from build123d import *

# Parameters (mm, degrees)
SKETCH_2_W          = 350
SKETCH_2_H          = 200
EXTRUDE_1_DEPTH     = 150
SHELL_1_T           = -20
CUT_EXTRUDE_1_REACH = 426.016
SKETCH_3_R          = 5
CUT_EXTRUDE_2_REACH = 426.016
SKETCH_4_R          = 7.5
CUT_EXTRUDE_3_REACH = 424.637


with BuildPart() as part:
    # 草图2 → 凸台-拉伸1 (new body)
    with BuildSketch(Plane(origin=(0, 0, 0), x_dir=(1, 0, 0), z_dir=(0, 1, 0))):
        with Locations((165.766338514, -86.518854231)):
            Rectangle(SKETCH_2_W, SKETCH_2_H)
    extrude(amount=EXTRUDE_1_DEPTH)

    # 抽壳1
    shell_1_openings = [part.faces().sort_by_distance(p)[0] for p in [
        (165.766338514, 150, 86.518854231),
    ]]
    offset(amount=SHELL_1_T, openings=shell_1_openings, kind=Kind.INTERSECTION)

    # 草图3 → 切除-拉伸1 (cut, up to next)
    with BuildSketch(Plane.ZY.offset(9.233661486), mode=Mode.PRIVATE) as cut_extrude_1_sk1:
        with Locations((55.039711013, 97.66717145)):
            Circle(SKETCH_3_R)
    cut_extrude_1_tool1 = extrude(cut_extrude_1_sk1.sketch, amount=-CUT_EXTRUDE_1_REACH, mode=Mode.PRIVATE) & part.part
    # 草图3 → 切除-拉伸1 (cut, up to next)
    with BuildSketch(Plane.ZY.offset(9.233661486), mode=Mode.PRIVATE) as cut_extrude_1_sk2:
        with Locations((112.314263257, 97.66717145)):
            Circle(SKETCH_3_R)
    cut_extrude_1_tool2 = extrude(cut_extrude_1_sk2.sketch, amount=-CUT_EXTRUDE_1_REACH, mode=Mode.PRIVATE) & part.part
    # 草图3 → 切除-拉伸1 (cut, up to next)
    with BuildSketch(Plane.ZY.offset(9.233661486), mode=Mode.PRIVATE) as cut_extrude_1_sk3:
        with Locations((55.039711013, 62.690345652)):
            Circle(SKETCH_3_R)
    cut_extrude_1_tool3 = extrude(cut_extrude_1_sk3.sketch, amount=-CUT_EXTRUDE_1_REACH, mode=Mode.PRIVATE) & part.part
    # 草图3 → 切除-拉伸1 (cut, up to next)
    with BuildSketch(Plane.ZY.offset(9.233661486), mode=Mode.PRIVATE) as cut_extrude_1_sk4:
        with Locations((112.314263257, 62.690345652)):
            Circle(SKETCH_3_R)
    cut_extrude_1_tool4 = extrude(cut_extrude_1_sk4.sketch, amount=-CUT_EXTRUDE_1_REACH, mode=Mode.PRIVATE) & part.part
    add(cut_extrude_1_tool1.solids().sort_by_distance((-9.233661, 97.667171, 55.039711))[0], mode=Mode.SUBTRACT)
    add(cut_extrude_1_tool2.solids().sort_by_distance((-9.233661, 97.667171, 112.314263))[0], mode=Mode.SUBTRACT)
    add(cut_extrude_1_tool3.solids().sort_by_distance((-9.233661, 62.690346, 55.039711))[0], mode=Mode.SUBTRACT)
    add(cut_extrude_1_tool4.solids().sort_by_distance((-9.233661, 62.690346, 112.314263))[0], mode=Mode.SUBTRACT)

    # 草图4 → 切除-拉伸2 (cut, up to next)
    with BuildSketch(Plane(origin=(340.766338514, 0, 0), x_dir=(0, 0, -1), z_dir=(1, 0, 0)), mode=Mode.PRIVATE) as cut_extrude_2_sk1:
        with Locations((-85.318851387, 90.981577925)):
            Circle(SKETCH_4_R)
    cut_extrude_2_tool1 = extrude(cut_extrude_2_sk1.sketch, amount=-CUT_EXTRUDE_2_REACH, mode=Mode.PRIVATE) & part.part
    add(cut_extrude_2_tool1.solids().sort_by_distance((340.766339, 90.981578, 85.318851))[0], mode=Mode.SUBTRACT)

    # 草图5 → 切除-拉伸3 (cut, up to next)
    with BuildSketch(Plane.XY.offset(186.518854231), mode=Mode.PRIVATE) as cut_extrude_3_sk1:
        with BuildLine():
            Line((242.364675661, 117.233767731), (272.364675661, 117.233767731))
            ThreePointArc((272.364675661, 117.233767731), (274.864675661, 114.733767731), (272.364675661, 112.233767731))
            Line((272.364675661, 112.233767731), (242.364675661, 112.233767731))
            ThreePointArc((242.364675661, 112.233767731), (239.864675661, 114.733767731), (242.364675661, 117.233767731))
        make_face()
    cut_extrude_3_tool1 = extrude(cut_extrude_3_sk1.sketch, amount=-CUT_EXTRUDE_3_REACH, mode=Mode.PRIVATE) & part.part
    add(cut_extrude_3_tool1.solids().sort_by_distance((257.364676, 114.733768, 186.518854))[0], mode=Mode.SUBTRACT)


solid = part.part
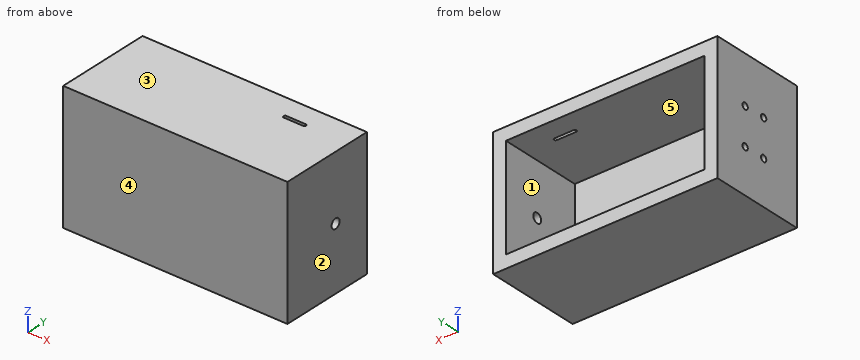
Geometry check sheet. Reference: the model listing, model coordinates, mm. Face numbers are marked on the shaded views. A direction names the side the tool comes from. Round coordinates to 2 decimals unless told otherwise and drop trailing zeros. Loops run counter-clockwise (first coordinate to the right, second up) from the corner with the lowest first, then second, coordinate; pieces in that order, holes last.
Item 1: Cross-section at C-C on z = 112. Record the boundary of the cut face in (x, y).
Item 2: Cross-section at B-B on x = 253.5. Record the boundary of the cut face in (y, z), then the cut area to 3 significant figures.
Item 3: Thickness scan on line 1 (X direction, y = 94.5, z = 108); line 2 (Z direction, x = 306, y = 137); line 3 (Y direction, x = 219, z = 68.5). Record the ranges inside material, lowest first.
Item 4: Access from +Z, -Z, +X, -X, +Y, -Y to the whole of each face (thin tool, end or side, straight path). Record for the marked faces 4 and 5.
Item 5: Gauge pin test, flat end, axial feed: pin 1 (8 mm diameter, centred on x = 147.5, z = 135.5, fed in from +Y). Record the tip position at first contact, or that the pin passes through.
Item 6: Cross-section at D-D on z = 157. Record the boundary of the cut face in (x, y), then the cut area to 3 significant figures.
Item 7: Cross-section at A-A on y = 78. Record the boundary of the cut face in (x, z).
Item 8: Mould release check, pull along X, two halves, no side actions. Record for the marked faces 1, 2 and 3: pulls with the +X half, pulls with the -X half, needs draft (parallel to the pull), parting line crosses it, or undercut.
Answer sheet:
1. outline: (-9.23, 0) - (340.77, 0) - (340.77, 150) - (320.77, 150) - (320.77, 20) - (10.77, 20) - (10.77, 57.7) - (-9.23, 57.7) - close; (-9.23, 67.68) - (10.77, 67.68) - (10.77, 92.68) - (-9.23, 92.68) - close; (-9.23, 102.66) - (10.77, 102.66) - (10.77, 150) - (-9.23, 150) - close
2. outline: (0, -13.48) - (150, -13.48) - (150, 6.52) - (20, 6.52) - (20, 166.52) - (112.23, 166.52) - (112.23, 186.52) - (0, 186.52) - close; (117.23, 166.52) - (150, 166.52) - (150, 186.52) - (117.23, 186.52) - close
2. area: 9,100 mm2
3. line 1: x = -9.23 to 10.77, 320.77 to 340.77
3. line 2: z = -13.48 to 6.52, 166.52 to 186.52
3. line 3: y = 0 to 20
4. face 4: +Z, -Z, +X, -X, -Y
4. face 5: +Y
5. pin 1: stops at y = 20
6. outline: (-9.23, 0) - (340.77, 0) - (340.77, 150) - (320.77, 150) - (320.77, 20) - (10.77, 20) - (10.77, 150) - (-9.23, 150) - close
6. area: 12,200 mm2
7. outline: (-9.23, -13.48) - (340.77, -13.48) - (340.77, 186.52) - (-9.23, 186.52) - close; hole (10.77, 6.52) - (320.77, 6.52) - (320.77, 166.52) - (10.77, 166.52) - close
8. face 1: undercut
8. face 2: pulls with the +X half
8. face 3: needs draft
